The drawing under review shows one solid part. Ordinate dimensions are in mm from its lowest x, y, z. Coordinates: 2 decimals unless noted, no trailing zeros. Loops run counter-clockwise (first coordinate to the right, second up) from the corner with the lowest first, then second, coordinate; pieces in that order, holes last. Notation, with made-up numbers: (37, -10.75) - (49, -10.75) arc R14 cw to (49, 11.25) - close; hole circle Ø8 at (57.25, 13). An arc over 180 degrees is marked (long way). Answer as a JSON object with one key per item and string values. Group by question number.
Item 1: To check wall thickness, follow line 1 (Y direction, x = 21, z = 0.95); line 2 (Y direction, x = 5, z = 1.95); line 3 (X direction, y = 44, z = 2.85). State the ranges of each line that lie inside material, in increasing order.
Item 2: We need section A-A (y = 25). Give the boundary of the cut face in (x, z).
Item 3: We need section D-D (y = 5). Give the boundary of the cut face in (x, z).
Item 4: We need section C-C (x = 60). Give the boundary of the cut face in (y, z).
Item 5: We need section B-B (x = 48). Give the boundary of the cut face in (y, z).
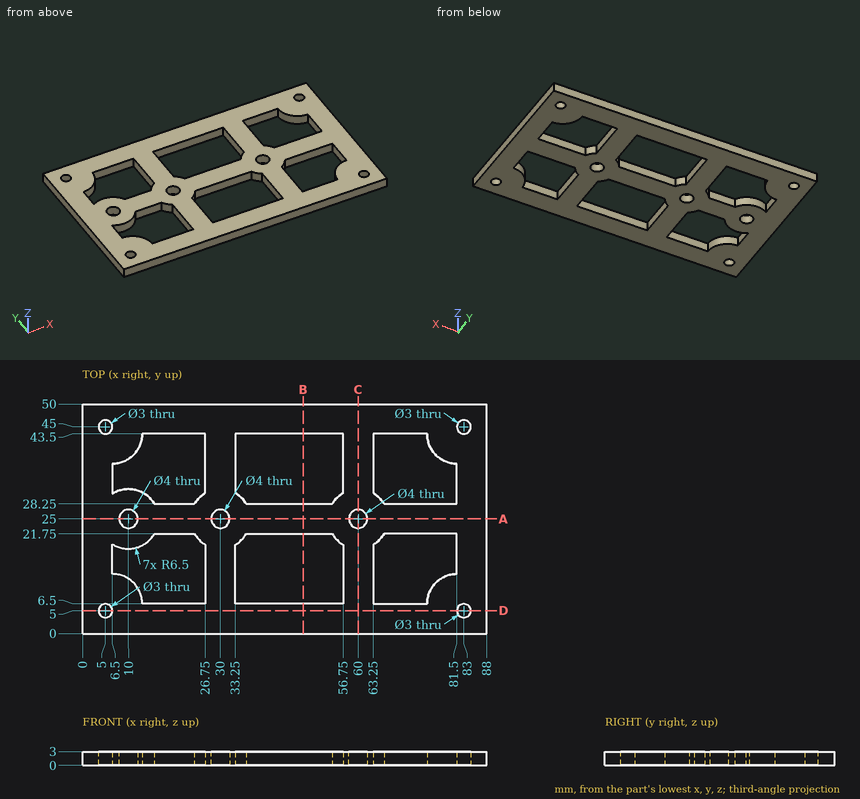
Check sheet entries:
{
 "1": {"line 1": "y = 0 to 6.5, 21.75 to 28.25, 43.5 to 50", "line 2": "y = 0 to 3.5, 6.5 to 43.5, 46.5 to 50", "line 3": "x = 0 to 3.88, 6.12 to 81.88, 84.12 to 88"},
 "2": {"outline": "(0, 0) - (8, 0) - (8, 3) - (0, 3) - close; (12, 0) - (28, 0) - (28, 3) - (12, 3) - close; (32, 0) - (58, 0) - (58, 3) - (32, 3) - close; (62, 0) - (88, 0) - (88, 3) - (62, 3) - close"},
 "3": {"outline": "(0, 0) - (3.5, 0) - (3.5, 3) - (0, 3) - close; (6.5, 0) - (81.5, 0) - (81.5, 3) - (6.5, 3) - close; (84.5, 0) - (88, 0) - (88, 3) - (84.5, 3) - close"},
 "4": {"outline": "(0, 0) - (23, 0) - (23, 3) - (0, 3) - close; (27, 0) - (50, 0) - (50, 3) - (27, 3) - close"},
 "5": {"outline": "(0, 0) - (6.5, 0) - (6.5, 3) - (0, 3) - close; (21.75, 0) - (28.25, 0) - (28.25, 3) - (21.75, 3) - close; (43.5, 0) - (50, 0) - (50, 3) - (43.5, 3) - close"}
}
